```python
from build123d import *

# Parameters (mm, degrees)
BOSS_EXTRUDE1_DEPTH      = 1.016
BOSS_EXTRUDE1_DEPTH_BACK = 1.016
SKETCH3_W                = 123.952
SKETCH3_H                = 174.752
SKETCH3_R                = 3.175


with BuildPart() as part:
    # Sketch3 → Boss-Extrude1 (new, two sides: drawn at the far end of the back side and taken through both)
    with BuildSketch(Plane.XY.offset(-BOSS_EXTRUDE1_DEPTH_BACK)):
        Rectangle(SKETCH3_W, SKETCH3_H)
        with Locations((-53.975, 79.375)):
            Circle(SKETCH3_R, mode=Mode.SUBTRACT)
        with Locations((53.975, 79.375)):
            Circle(SKETCH3_R, mode=Mode.SUBTRACT)
        with Locations((-53.975, -79.375)):
            Circle(SKETCH3_R, mode=Mode.SUBTRACT)
        with Locations((53.975, -79.375)):
            Circle(SKETCH3_R, mode=Mode.SUBTRACT)
    extrude(amount=BOSS_EXTRUDE1_DEPTH + BOSS_EXTRUDE1_DEPTH_BACK)


solid = part.part
```
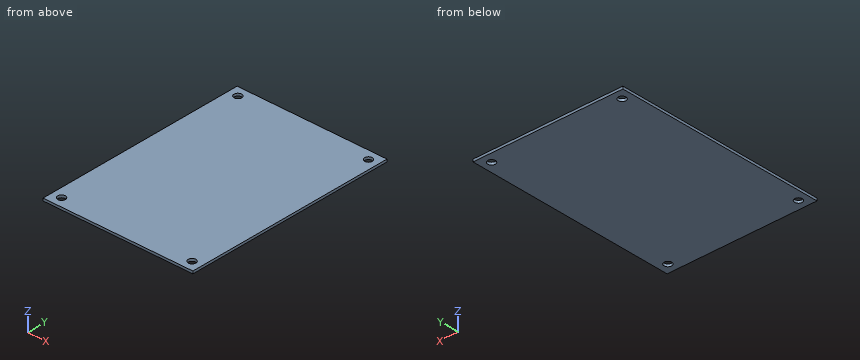
CAD build for the part. Positions are in the model's coordinates, mm. Coordinates: 2 decimals unless noted, no trailing zeros. Order: outer loops, then holes, each group sorted by start corner. A loop starts at its lowest first (then second) coordinate and runs counter-clockwise, first axis right, second up. Notation, with made-up numbers: (54, 50.25) - (81, 50.25) arc R13 cw to (81, 73.25) - close; hole circle Ø6 at (26, 80.5). An arc over 180 degrees is marked (long way). Use a Markdown table: item, result. Add a question column.
(1) Saw through at A-A (x = -53.5). Give the cut face in (y, z), then the cut area to 3 significant figures.
(2) Flat gauge pins, fed straight in: pin 1 (5 mm diameter, centred on x = 53.975, y = 79.375, fed in from +Z); pin 2 (7.5 mm diameter, centred on x = -53.975, y = -79.375, fed in from -Z). Where does each tip first touch, or does it go through?
(3) Drill centre lines: line 1 along Y through (x, z) = (-54, 0.1); line 2 along Y through (x, z) = (-52.5, 0.8). Where is each one in solid material? Low to high. Write a range as [from, to].
Solved:
| question | item | result |
|---|---|---|
| 1 | outline | (-87.38, -1.02) - (-82.51, -1.02) - (-82.51, 1.02) - (-87.38, 1.02) - close; (-76.24, -1.02) - (76.24, -1.02) - (76.24, 1.02) - (-76.24, 1.02) - close; (82.51, -1.02) - (87.38, -1.02) - (87.38, 1.02) - (82.51, 1.02) - close |
| 1 | area | 330 mm² |
| 2 | pin 1 | passes through |
| 2 | pin 2 | stops at z = -1.02 |
| 3 | line 1 | y = [-87.38, -82.55], [-76.2, 76.2], [82.55, 87.38] |
| 3 | line 2 | y = [-87.38, -82.19], [-76.56, 76.56], [82.19, 87.38] |
